Work out the finished part from the listing and answer in its coordinate system (mm). Face numbers are marked on the shaded views. Coordinates: 2 decimals unless noted, no trailing zeros. Loops run counter-clockwise (first coordinate to the right, second up) from the corner with the lowest first, then second, coordinate; pieces in that order, holes last. Notation, with made-up numbers: (49.5, 64) - (93.5, 64) arc R15 cw to (93.5, 84) - close; hole circle Ø7 at (-23.75, -31). An arc over 180 degrees is marked (long way). Write each question's results on one line, items separated by ' | '. Start each with the question number.
1. A cutting plane is placed at D-D on z = 6. Determine the outline of the cut face in (x, y).
2. A cutting plane is placed at A-A on y = 0. Determine the outline of the cut face in (x, z).
3. Each of these flat-tipped pins is pushed along its axis until it touches: P1, Ø10, axis at x = 4, y = -29, coming from the -Z side; P2, Ø10, axis at x = -5.5, z = 69, coming from the -Y side; P3, Ø12, axis at y = -12.5, z = 12.5, coming from the -X side. Where does it stop, or does it pass through?
4. A cutting plane is placed at B-B on z = 69.5. Determine the outline of the cut face in (x, y), then the cut area to 3 significant figures.
5. A cutting plane is placed at C-C on x = -3.25. Determine the outline of the cut face in (y, z).
6. Determine the mould class of the marked faces 1, 2 and 3 for opening direction X: released by +X, released by -X, zero draft, split by the parting line, or undercut.
7. Find the intervals of material crossed by line 1 along X through (y, z) = (-5, -25); line 2 along Z through (x, y) = (5, 4); line 3 along Y through (x, z) = (-7.75, 84.5), in increasing order. Write a range as [from, to].
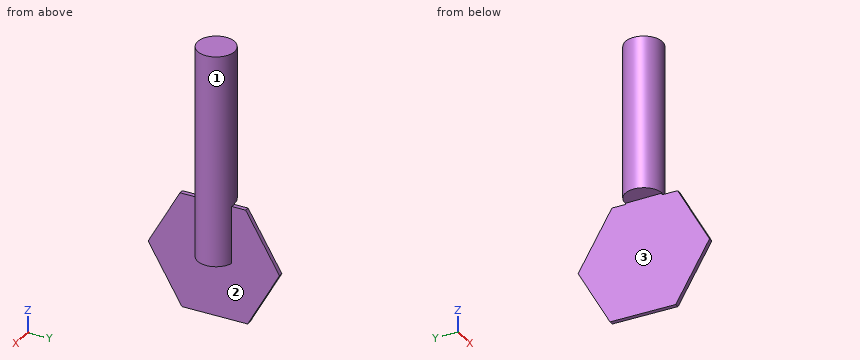
from build123d import *

# Parameters (mm, degrees)
F0_R          = 11.060744
F1_DEPTH      = 127
F3_DEPTH      = 2.54
F4_W          = 12.080216
F4_H          = 35.164498
F5_DEPTH      = 39.601066
F5_DEPTH_BACK = 25.4


with BuildPart() as f1:
    # F0 (on Top) → F1 (new body)
    with BuildSketch(Plane.XY):
        Circle(F0_R)
    extrude(amount=F1_DEPTH)

    # F2 (on Right) → F3 (join)
    with BuildSketch(Plane.YZ):
        Polygon((20.383448, -33.957828), (39.600066, 0.67367), (19.216617, 34.631498), (-20.383448, 33.957828), (-39.600066, -0.67367), (-19.216617, -34.631498), align=None)
    extrude(amount=F3_DEPTH)

    # F4 (on Front) → F5 (cut, two sides)
    with BuildSketch(Plane.XZ) as f5_sk:
        with Locations((-6.040108, 17.582249)):
            Rectangle(F4_W, F4_H)
    extrude(amount=F5_DEPTH, mode=Mode.SUBTRACT)
    extrude(f5_sk.sketch, amount=-F5_DEPTH_BACK, mode=Mode.SUBTRACT)


solid = f1.part
Values:
1) outline: (0, -35.9) - (2.54, -35.9) - (2.54, -10.77) arc R11.06 ccw to (2.54, 10.77) - (2.54, 36.4) - (0, 36.4) - close
2) outline: (-11.06, 35.16) - (0, 35.16) - (0, -34.3) - (2.54, -34.3) - (2.54, 0) - (11.06, 0) - (11.06, 127) - (-11.06, 127) - close
3) P1: z = -26.3 | P2: y = -11.05 | P3: x = 0
4) outline: circle Ø22.12 at (0, 0) | area: 384 mm^2
5) outline: (-10.57, 35.16) - (10.57, 35.16) - (10.57, 127) - (-10.57, 127) - close
6) face 1: split by the parting line | face 2: released by +X | face 3: released by -X
7) line 1: [0, 2.54] | line 2: [0, 127] | line 3: [-7.89, 7.89]
